Study the drawing (mm; zero at the part's minimum x, y, z) and answer. Coordinates: 2 decimals unless noted, no trailing zeros. Order: outer loops, then holes, each group sorted by start corner. A loop starts at its lowest first (then second) coordinate and runs counter-clockwise, first axis right, second up. Notation, with made-up numbers: (63, 11.5) -> (99, 11.5) arc R37 cw to (99, 48.5) -> close; hole circle Ø10 at (42.5, 20). An arc over 180 degrees is marked (long way). Answer as CSV lines item,"result". Start each with the question number.
Item 1: Section D-D (z = 3.75) is taken. Write down the section's boundary in (x, y), then the cut area to 3 significant figures.
Item 2: Straight lines are drawn through the part: L1, parallel to Y at x = 35.5, z = 10; L2, parallel to Y at x = 5, z = 11.75 (1 decimal); L3, parallel to Y at x = 8, z = 3.75. For each, find the intervals that lie inside material, in ascending order.
Item 3: Section C-C (x = 17.5) is taken. Write down the section's boundary in (y, z), then the cut area to 3 significant figures.
Item 4: Section A-A (z = 10) is taken. Write down the section's boundary in (x, y), then the cut area to 3 significant figures.
Item 5: Section B-B (y = 10.5) is taken. Write down the section's boundary in (x, z).
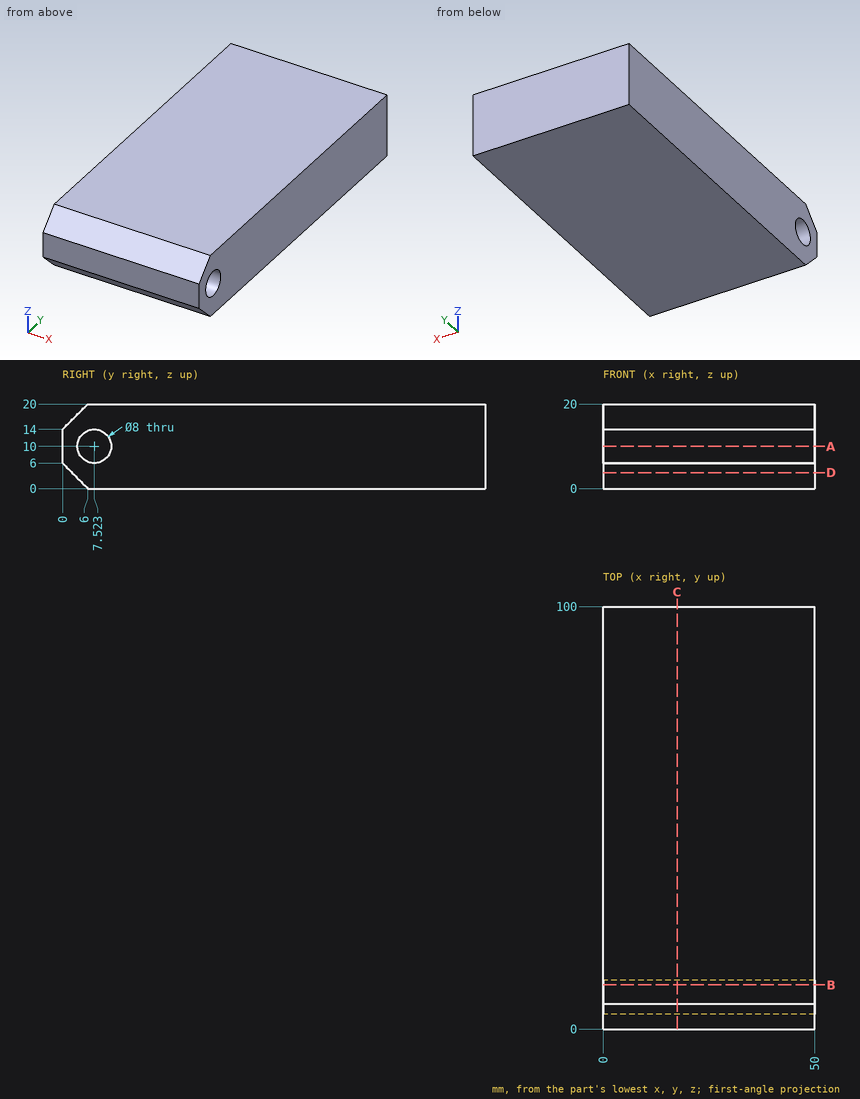
Checked values:
1,outline,"(0, 2.25) -> (50, 2.25) -> (50, 100) -> (0, 100) -> close"
1,area,"4,890 mm^2"
2,L1,"y = 0 to 3.52, 11.52 to 100"
2,L2,"y = 0 to 3.9, 11.1 to 100"
2,L3,"y = 2.25 to 100"
3,outline,"(0, 6) -> (6, 0) -> (100, 0) -> (100, 20) -> (6, 20) -> (0, 14) -> close; hole circle Ø8 at (7.52, 10)"
3,area,"1,910 mm^2"
4,outline,"(0, 0) -> (50, 0) -> (50, 3.52) -> (0, 3.52) -> close; (0, 11.52) -> (50, 11.52) -> (50, 100) -> (0, 100) -> close"
4,area,"4,600 mm^2"
5,outline,"(0, 0) -> (50, 0) -> (50, 7.33) -> (0, 7.33) -> close; (0, 12.67) -> (50, 12.67) -> (50, 20) -> (0, 20) -> close"
